Could you check a few things on this model? Use its own coordinates, in mm. Face numbers are marked on the shaded views. A direction names the side the tool comes from. Give positions to 0.01 mm unless a question says otherwise; leave off trailing zeros. Write each loop counter-clockwise with the first axis right and the second up, starting at its lowest first coordinate (ties: lowest second). Pieces come first, ordered by that corner, then holes. Notation, with made-up numbers: (61, 41.25) - (100, 41.25) arc R14 ccw to (100, 56.25) - close; hole circle Ø2 at (-14, 28.5). An arc over 180 degrees is marked (long way). Use one line per item in the form item = value.
```python
from build123d import *

# Parameters (mm, degrees)
F0_R     = 4.0581916303
F1_DEPTH = 1.905
F2_R     = 1.27


with BuildPart() as f1:
    # F0 (on Front) → F1 (new body, symmetric)
    with BuildSketch(Plane.XZ):
        Circle(F0_R)
        Polygon((-1.8276859231, 3.5948536131), (2.1993915903, 3.3802492461), (4.0270775134, -0.2146043671), (1.8276859231, -3.5948536131), (-2.1993915903, -3.3802492461), (-4.0270775134, 0.2146043671), align=None, mode=Mode.SUBTRACT)
    extrude(amount=F1_DEPTH, both=True)

    # F2
    f2_edges = [f1.edges().sort_by_distance(p)[0] for p in [
        (-1.827686, 0, 3.594854),
        (2.199392, 0, 3.380249),
        (4.027078, 0, -0.214604),
        (-4.027078, 0, 0.214604),
        (-2.199392, 0, -3.380249),
        (1.827686, 0, -3.594854),
    ]]
    fillet(f2_edges, radius=F2_R)


solid = f1.part
```
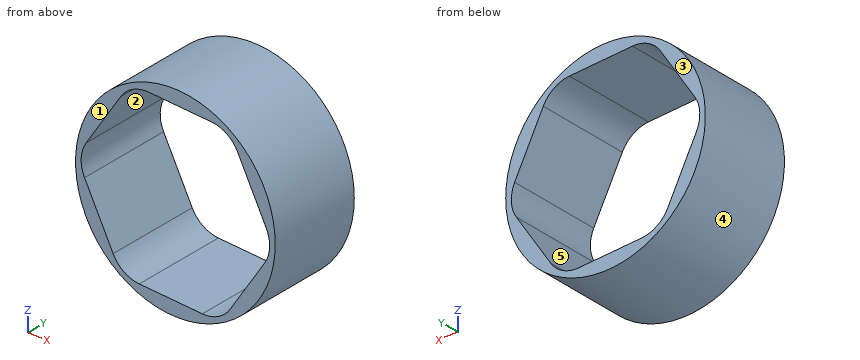
1. Which directions (+Z, -Z, +X, -X, +Y, -Y) give clear straight access to the entire face, cutting with the end or side of a thin tool? Please do the marked faces 1 and 2.
Response values:
face_1 = +Z, -Z, +X, -X, -Y
face_2 = +Y, -Y
2. Imagine slicing it at B-B, the plane x = 0. List the corners of the cut face in (y, z) for me (3 decimals), and give its area (3 significant figures).
Response values:
outline = (-1.905, -4.058) - (1.905, -4.058) - (1.905, -3.497) - (-1.905, -3.497) - close; (-1.905, 3.497) - (1.905, 3.497) - (1.905, 4.058) - (-1.905, 4.058) - close
area = 4.27 mm²
3. If we mould it in two halves opening along Z, with no side actions, what happens to the marked faces 3, 4 and 5? For each: pulls with the +Z half, pulls with the -Z half, needs draft (parallel to the pull), parting line crosses it, or undercut.
Response values:
face_3 = needs draft
face_4 = parting line crosses it
face_5 = undercut
4. Imagine slicing it at A-A, the plane y = -0.1. List the corners of the cut face in (x, z) for me, and give its area (3 significant figures).
Response values:
outline = circle Ø8.12 at (0, 0); hole (-3.69, -0.44) - (-2.53, -2.73) arc R1.27 ccw to (-1.47, -3.42) - (1.1, -3.56) arc R1.27 ccw to (2.23, -2.98) - (3.63, -0.83) arc R1.27 ccw to (3.69, 0.44) - (2.53, 2.73) arc R1.27 ccw to (1.47, 3.42) - (-1.1, 3.56) arc R1.27 ccw to (-2.23, 2.98) - (-3.63, 0.83) arc R1.27 ccw to start
area = 10.0 mm²
5. Imagine slicing it at C-C, the plane z = 0. List the corners of the cut face in (x, y) for me (3 decimals).
Response values:
outline = (-4.058, -1.905) - (-3.825, -1.905) - (-3.825, 1.905) - (-4.058, 1.905) - close; (3.825, -1.905) - (4.058, -1.905) - (4.058, 1.905) - (3.825, 1.905) - close
6. For pin 1 (3 mm diameter, centred on x = 2, z = 2.5, fed in from +Y) (3 decimals); pin 2 (1.5 mm diameter, centred on x = 3, y = 0, fed in from +Z), each with a flat end and sliding along its axis, tell me the tip position at first contact or that it passes through.
Response values:
pin_1 = 1.905
pin_2 = 3.38
7. If I drill on line 1 (X direction, y = 0.05, z = -3.25); line 2 (Z direction, x = -0.75, y = -0.55); line 3 (X direction, y = 0.2, z = -2.5), over which ranges is the centre line in solid material (lowest first)? Write a range as from..to.
Response values:
line_1 = -2.43..-2.04, 1.99..2.43
line_2 = -3.99..-3.46, 3.54..3.99
line_3 = -3.2..-2.65, 2.54..3.2
